Build history of the part. All positions in model axes, mm. Give positions to 0.01 mm unless a question says otherwise; leave off trailing zeros. Write each loop counter-clockwise with the first axis right and the second up, starting at its lowest first coordinate (ties: lowest second). Pieces come first, ordered by that corner, then holes. Notation, with made-up numbers: (77, 87) -> (82, 87) arc R19 cw to (82, 120) -> close; hole circle Ø10 at (40.5, 50). An arc over 180 degrees is marked (long way). Put each result on its own line as item: value.
from build123d import *

# Parameters (mm, degrees)
F0_W     = 45
F0_H     = 10
F0_W_2   = 3
F0_H_2   = 2
F1_DEPTH = 15
F2_DEPTH = 5


with BuildPart() as f1:
    # F0 (on Top) → F1 (new body)
    with BuildSketch(Plane.XY):
        Rectangle(F0_W, F0_H)
        with Locations((-13.5, 0)):
            Rectangle(F0_W_2, F0_H_2, mode=Mode.SUBTRACT)
        with Locations((-4.5, 0)):
            Rectangle(F0_W_2, F0_H_2, mode=Mode.SUBTRACT)
        Polygon((3, -1), (3, 0), (3, 1), (6, 1), (6, 0), (6, -1), align=None, mode=Mode.SUBTRACT)
        Polygon((12, -1), (12, 0), (12, 1), (15, 1), (15, -1), align=None, mode=Mode.SUBTRACT)
    extrude(amount=F1_DEPTH)

    # F0 (on Top) → F2 (join)
    with BuildSketch(Plane.XY):
        with Locations((-13.5, 0)):
            Rectangle(F0_W_2, F0_H_2)
        with Locations((-4.5, 0)):
            Rectangle(F0_W_2, F0_H_2)
        Polygon((3, 1), (3, 0), (4.5, 0), (6, 0), (6, 1), align=None)
        Polygon((4.5, 0), (3, 0), (3, -1), (6, -1), (6, 0), align=None)
        Polygon((12, 1), (12, 0), (12, -1), (15, -1), (15, 1), align=None)
    extrude(amount=F2_DEPTH)


solid = f1.part
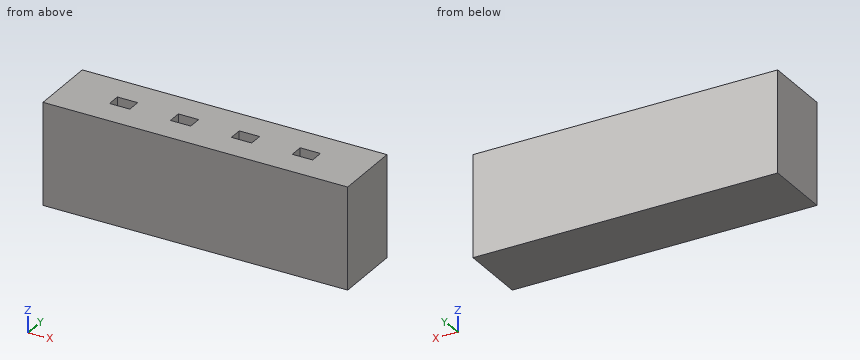
1) Slice it at C-C (x = -12.5). Write the cut outline in (y, z), plus the area to 3 significant figures.
Filled sheet:
outline: (-5, 0) -> (5, 0) -> (5, 15) -> (1, 15) -> (1, 5) -> (-1, 5) -> (-1, 15) -> (-5, 15) -> close
area: 130 mm2
2) Wall check: L1, parallel to X at y = 0.5, z = 13.5; L2, parallel to Y at x = -14.5, z = 6; L3, parallel to Z at x = 5, y = 0.25. Give the ranges that are in metal, low to high.
Filled sheet:
L1: -22.5 to -15, -12 to -6, -3 to 3, 6 to 12, 15 to 22.5
L2: -5 to -1, 1 to 5
L3: 0 to 5
3) Pin check, flat tip, straight feed: pin 1 (1.6 mm diameter, centred on x = 13.5, y = 0, fed in from +Z). Stop position of the tip, or through.
Filled sheet:
pin 1: z = 5
4) Slice it at A-A (z = 7.25). Write the cut outline in (x, y), plus the area to 3 significant figures.
Filled sheet:
outline: (-22.5, -5) -> (22.5, -5) -> (22.5, 5) -> (-22.5, 5) -> close; hole (-15, -1) -> (-12, -1) -> (-12, 1) -> (-15, 1) -> close; hole (-6, -1) -> (-3, -1) -> (-3, 1) -> (-6, 1) -> close; hole (3, -1) -> (6, -1) -> (6, 1) -> (3, 1) -> close; hole (12, -1) -> (15, -1) -> (15, 1) -> (12, 1) -> close
area: 426 mm2
5) Slice it at B-B (y = 0). Write the cut outline in (x, z), plus the area to 3 significant figures.
Filled sheet:
outline: (-22.5, 0) -> (22.5, 0) -> (22.5, 15) -> (15, 15) -> (15, 5) -> (12, 5) -> (12, 15) -> (6, 15) -> (6, 5) -> (3, 5) -> (3, 15) -> (-3, 15) -> (-3, 5) -> (-6, 5) -> (-6, 15) -> (-12, 15) -> (-12, 5) -> (-15, 5) -> (-15, 15) -> (-22.5, 15) -> close
area: 555 mm2
